Can you work these out from the drawing? Everything is in mm from the part's minimum corner. A direction names the side the tool comes from. Round coordinates to 2 decimals unless told otherwise and drop trailing zeros. Write each loop counter-clockwise with the first axis right and the second up, starting at its lowest first coordinate (ties: lowest second). Pieces come first, ordered by that corner, then holes. Notation, with made-up numbers: (8, 20) -> (30, 20) arc R18 cw to (30, 53) -> close; hole circle Ø6 at (12, -15). An arc over 180 degrees is marked (long way). Put each result on its own line as item: value. Start each with the question number.
1. Suppose I cut it at C-C (z = 28.5). Please give me the cut outline in (x, y).
2. Which directions (+Z, -Z, +X, -X, +Y, -Y) give clear straight access to the entire face, cutting with the end or side of a thin tool? Please do the marked faces 5, 6 and 7.
3. Suppose I cut it at D-D (y = 5). Please give me the cut outline in (x, z).
4. We'd pull the mould along Y, two halves only. Please class the marked faces 1, 2, 3 and 4: +Y half, -Y half, draft (parallel to the pull), parting line (faces both ways), or undercut.
5. I need wall thicknesses on probe 1 along Y at (x, z) = (10.5, 30.55); probe 2 along Y at (x, z) = (1.4, 4); probe 3 along Z at (x, y) = (3.75, 21.25). Which ranges of each line are inside material? Lowest first, please. Write a range as from..to.
6. Suppose I cut it at A-A (x = 10.5). Please give me the cut outline in (y, z), then the cut area to 3 significant figures.
7. For pin 1 (9.5 mm diameter, centred on y = 15, z = 12.5, fed in from +X); pin 2 (5 mm diameter, centred on x = 10.5, y = 5, fed in from +Z); pin 3 (3 mm diameter, centred on y = 16.5, z = 7.5, fed in from +X); pin 4 (3.5 mm diameter, centred on x = 6.5, y = 22, fed in from -Z), each with a flat end and sliding along its axis, tell me the tip position at first contact or that it passes through.
8. Suppose I cut it at B-B (y = 15). Please give me the cut outline in (x, z), then the cut area to 3 significant figures.
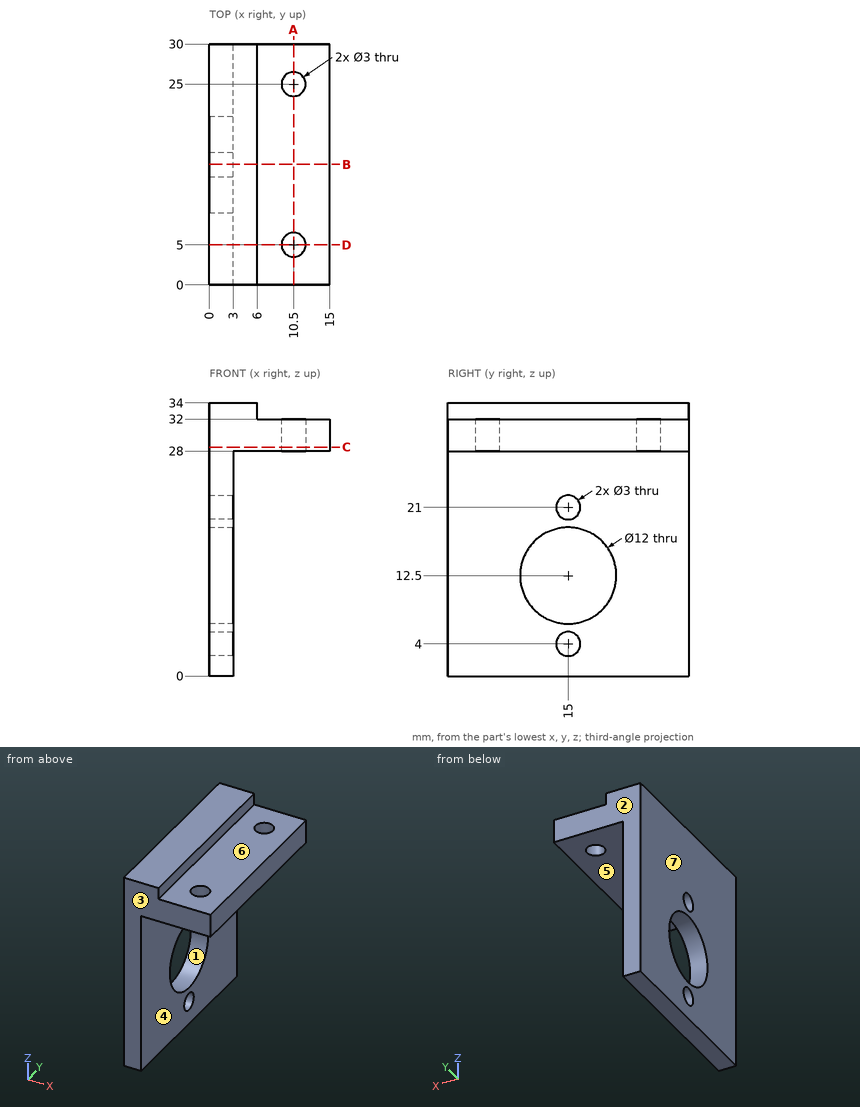
Verdict:
1. outline: (0, 0) -> (15, 0) -> (15, 30) -> (0, 30) -> close; hole circle Ø3 at (10.5, 5); hole circle Ø3 at (10.5, 25)
2. face 5: -Z, +X, +Y, -Y
2. face 6: +Z, +X, +Y, -Y
2. face 7: +Z, -Z, -X, +Y, -Y
3. outline: (0, 0) -> (3, 0) -> (3, 28) -> (9, 28) -> (9, 32) -> (6, 32) -> (6, 34) -> (0, 34) -> close; (12, 28) -> (15, 28) -> (15, 32) -> (12, 32) -> close
4. face 1: undercut
4. face 2: +Y half
4. face 3: -Y half
4. face 4: draft
5. probe 1: y = 0..3.5, 6.5..23.5, 26.5..30
5. probe 2: y = 0..13.5, 16.5..30
5. probe 3: z = 28..34
6. outline: (0, 28) -> (3.5, 28) -> (3.5, 32) -> (0, 32) -> close; (6.5, 28) -> (23.5, 28) -> (23.5, 32) -> (6.5, 32) -> close; (26.5, 28) -> (30, 28) -> (30, 32) -> (26.5, 32) -> close
6. area: 96.0 mm^2
7. pin 1: passes through
7. pin 2: stops at z = 32
7. pin 3: stops at x = 3
7. pin 4: stops at z = 28
8. outline: (0, 0) -> (3, 0) -> (3, 2.5) -> (0, 2.5) -> close; (0, 5.5) -> (3, 5.5) -> (3, 6.5) -> (0, 6.5) -> close; (0, 18.5) -> (3, 18.5) -> (3, 19.5) -> (0, 19.5) -> close; (0, 22.5) -> (3, 22.5) -> (3, 28) -> (15, 28) -> (15, 32) -> (6, 32) -> (6, 34) -> (0, 34) -> close
8. area: 102 mm^2
